Source: three-view drawing plus pictorial views. Frame: mm from the lowest corner of the part. A direction names the side the tool comes from. Coordinates: 2 decimals unless noted, no trailing zeros. Order: outer loops, then holes, each group sorted by start corner. A loop starts at its lowest first (then second) coordinate and runs counter-clockwise, first axis right, second up. Notation, with made-up numbers: (24, 88.5) - (29, 88.5) arc R15 ccw to (29, 100.5) - close; hole circle Ø3 at (82, 0.5). An arc over 180 degrees is marked (long way). One line per question, with ' | ' between items.
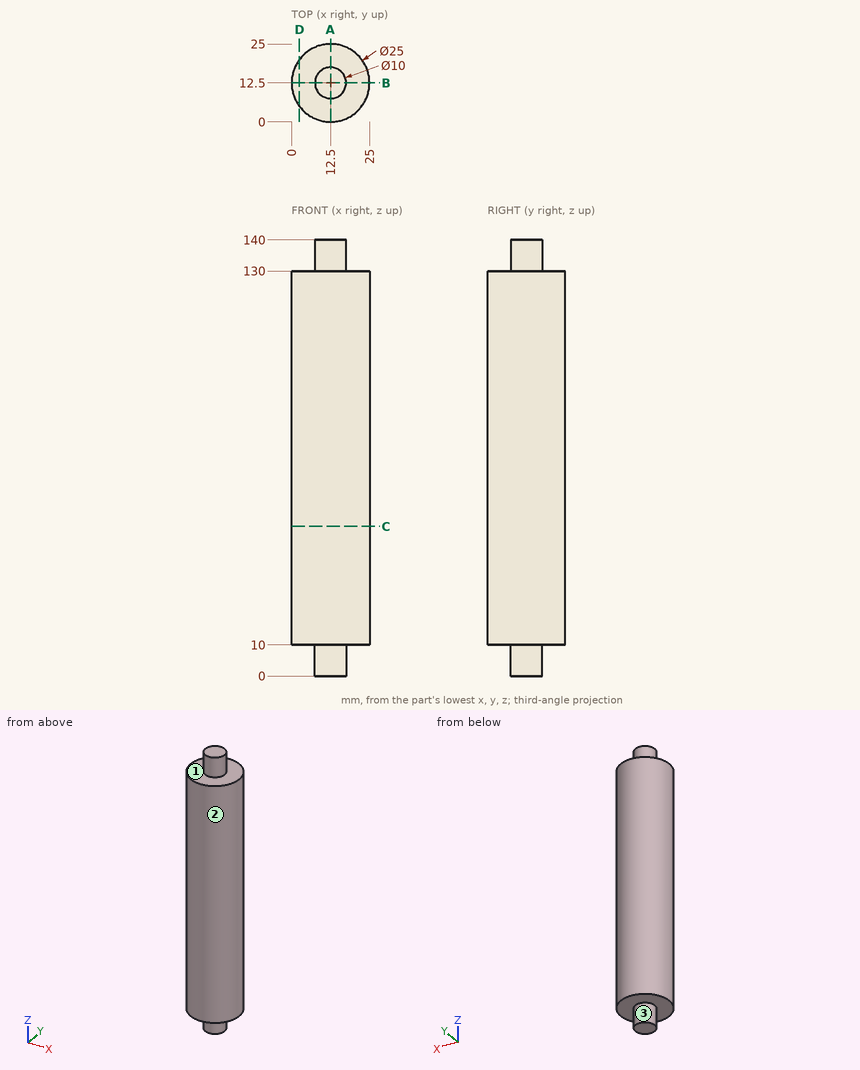
Item 1: Contact query for flat-ended pins moving along their axis: P1, Ø1, axis at x = 17.5, y = 9.5, coming from the -Z side; P2, Ø3, axis at x = 4.5, z = 38.5, coming from the +Y side; P3, Ø1.5, axis at x = 17.5, z = 16.5, coming from the -Y side. Output: stop coordinate, or through.
Data:
P1: z = 10 | P2: y = 23.18 | P3: y = 0.74
Item 2: Section D-D on x = 2.5. Return the cut outline in (y, z).
Data:
outline: (5, 10) - (20, 10) - (20, 130) - (5, 130) - close
Item 3: Section A-A on x = 12.5. Return the cut outline in (y, z), and give its area (3 significant figures).
Data:
outline: (0, 10) - (7.5, 10) - (7.5, 0) - (17.5, 0) - (17.5, 10) - (25, 10) - (25, 130) - (17.5, 130) - (17.5, 140) - (7.5, 140) - (7.5, 130) - (0, 130) - close | area: 3,200 mm^2
Item 4: Access query for the marked faces 1, 2 and 3. Directions: +Z, -Z, +X, -X, +Y, -Y. A direction counts if a zero-diameter tool reaches every point of the face in a straight line with its end or side. Return the directions, or none.
Data:
face 1: +Z | face 2: +Z, -Z | face 3: -Z
Item 5: Section C-C on z = 48. Return the cut outline in (x, y), and give its area (3 significant figures).
Data:
outline: circle Ø25 at (12.5, 12.5) | area: 491 mm^2
Item 6: Ray query, line 1 (Z direction, x = 1.25, y = 13.5); line 2 (Y direction, x = 12, z = 121). Return the intervals inside material, ascending.
Data:
line 1: 10 to 130 | line 2: 0.01 to 24.99
